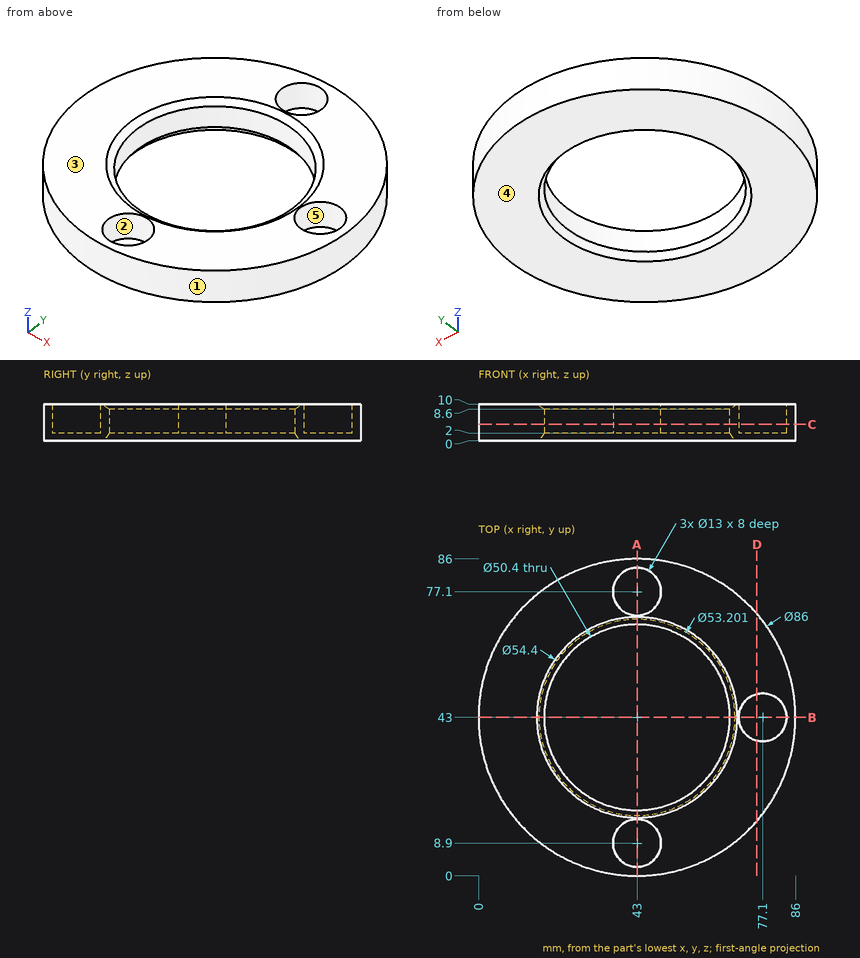
Check sheet for the drawn part. Datum: minimum x, y, z corner. Units: mm. A direction names the side the tool comes from. Give positions to 0.01 mm unless a question says otherwise; leave off trailing zeros. Order: outer loops, then holes, each group sorted by start corner. A loop starts at its lowest first (then second) coordinate and runs counter-clockwise, first axis right, second up.
1. Sectioned sample at A-A (x = 43). Record the boundary of the cut face in (y, z).
Completed:
outline: (0, 0) - (16.4, 0) - (17.8, 2) - (17.8, 8.6) - (15.8, 10) - (15.4, 10) - (15.4, 2) - (2.4, 2) - (2.4, 10) - (0, 10) - close; (68.2, 2) - (69.6, 0) - (86, 0) - (86, 10) - (83.6, 10) - (83.6, 2) - (70.6, 2) - (70.6, 10) - (70.2, 10) - (68.2, 8.6) - close
2. Access from +Z, -Z, +X, -X, +Y, -Y to the whole of each face (thin tool, end or side, straight path). Record for the marked faces 4 and 5.
Completed:
face 4: -Z, +X, -X, +Y, -Y
face 5: +Z
3. Sectioned sample at B-B (y = 43). Record the boundary of the cut face in (x, z).
Completed:
outline: (0, 0) - (16.4, 0) - (17.8, 2) - (17.8, 8.6) - (15.8, 10) - (0, 10) - close; (68.2, 2) - (69.6, 0) - (86, 0) - (86, 10) - (83.6, 10) - (83.6, 2) - (70.6, 2) - (70.6, 10) - (70.2, 10) - (68.2, 8.6) - close
4. Sectioned sample at C-C (z = 4.5). Record the boundary of the cut face in (x, y).
Completed:
outline: circle Ø86 at (43, 43); hole circle Ø50.4 at (43, 43); hole circle Ø13 at (43, 8.9); hole circle Ø13 at (43, 77.1); hole circle Ø13 at (77.1, 43)
5. Depth check by flat-ended pin: pin 1 (2 mm diameter, centred on x = 55.5, z = 1.5, fed in from -Y); pin 2 (6.5 mm diameter, centred on x = 76, y = 45.5, fed in from +Z); pin 3 (2 mm diameter, centred on x = 74.5, z = 4, fed in from -Y). Enter the tip coordinate at first touch or a pass-through.
Completed:
pin 1: stops at y = 1.57
pin 2: stops at z = 2
pin 3: stops at y = 12.69
6. Draft check along X on the marked faces 1, 2 and 3. Enter one of: pulls with the +X half, pulls with the -X half, needs draft (parallel to the pull), parting line crosses it, or undercut.
Completed:
face 1: parting line crosses it
face 2: undercut
face 3: needs draft
7. Scan lines: line 1 (Y direction, x = 43, z = 7); line 2 (X direction, y = 28, z = 8); line 3 (X direction, y = 60, z = 6) (1 decimal). Record each from-to range of solid material in increasing order.
Completed:
line 1: y = 0 to 2.4, 15.4 to 17.8, 68.2 to 70.6, 83.6 to 86
line 2: x = 2.7 to 22.75, 63.25 to 83.3
line 3: x = 3.5 to 24.4, 61.6 to 82.5
8. Sectioned sample at D-D (x = 75.5). Record the boundary of the cut face in (y, z) (1 decimal), then the cut area to 3 significant figures.
Completed:
outline: (14.8, 0) - (71.2, 0) - (71.2, 10) - (49.3, 10) - (49.3, 2) - (36.7, 2) - (36.7, 10) - (14.8, 10) - close
area: 462 mm2
